```python
from build123d import *

# Parameters (mm, degrees)
DODANIE_WYCI_GNI_CIE1_DEPTH = 1.2
SZKIC3_R                    = 2.5
DODANIE_WYCI_GNI_CIE2_DEPTH = 8
SZKIC4_R                    = 1.5
WYTNIJ_WYCI_GNI_CIE1_DEPTH  = 706.226503642
SZKIC5_W                    = 5
SZKIC5_H                    = 5
DODANIE_WYCI_GNI_CIE3_DEPTH = 1
SZKIC6_W                    = 8
SZKIC6_H                    = 8
DODANIE_WYCI_GNI_CIE4_DEPTH = 3
SZKIC7_R                    = 2.5
DODANIE_WYCI_GNI_CIE5_DEPTH = 3
SZKIC8_W                    = 20.5
SZKIC8_H                    = 4
SZKIC8_H_2                  = 10
DODANIE_WYCI_GNI_CIE6_DEPTH = 2
SZKIC9_W                    = 0.66
SZKIC9_H                    = 0.66
DODANIE_WYCI_GNI_CIE7_DEPTH = 6
SZYK_LINIOWY1_COUNT         = 8
SZYK_LINIOWY1_PITCH         = 2.54
SZKIC10_W                   = 10
SZKIC10_H                   = 12
SZKIC10_W_2                 = 5
DODANIE_WYCI_GNI_CIE8_DEPTH = 2


with BuildPart() as part:
    # Szkic2 → Dodanie-wyciągnięcie1 (new body)
    with BuildSketch(Plane(origin=(0, 566.370308932, 0), x_dir=(1, 0, 0), z_dir=(0, 1, 0))):
        Polygon((-513.826446608, 398.472881439), (-513.826446608, 383.472881439), (-419.826446608, 383.472881439), (-419.826446608, 482.972881439), (-513.826446608, 482.972881439), (-513.826446608, 454.472881439), (-438.826446608, 454.472881439), (-438.826446608, 398.472881439), align=None)
    extrude(amount=DODANIE_WYCI_GNI_CIE1_DEPTH)

    # Szkic3 → Dodanie-wyciągnięcie2 (add)
    with BuildSketch(Plane(origin=(0, 567.570308932, 0), x_dir=(1, 0, 0), z_dir=(0, 1, 0))):
        with Locations(Location((-506.326446608, 461.972881439, 0), (0, 0, 180))):
            Circle(SZKIC3_R)
        with Locations(Location((-496.326446608, 461.972881439, 0), (0, 0, 180))):
            Circle(SZKIC3_R)
        with Locations(Location((-496.326446608, 390.972881439, 0), (0, 0, 180))):
            Circle(SZKIC3_R)
        with Locations(Location((-506.326446608, 390.972881439, 0), (0, 0, 180))):
            Circle(SZKIC3_R)
    extrude(amount=DODANIE_WYCI_GNI_CIE2_DEPTH)

    # Szkic4 → Wytnij-wyciągnięcie1 (cut, through all)
    with BuildSketch(Plane(origin=(0, 567.570308932, 0), x_dir=(1, 0, 0), z_dir=(0, 1, 0))):
        with Locations(Location((-434.826446608, 401.472881439, 0), (0, 0, 180))):
            Circle(SZKIC4_R)
        with Locations(Location((-434.826446608, 451.472881439, 0), (0, 0, 180))):
            Circle(SZKIC4_R)
    extrude(amount=-WYTNIJ_WYCI_GNI_CIE1_DEPTH, mode=Mode.SUBTRACT)

    # Szkic5 → Dodanie-wyciągnięcie3 (add)
    with BuildSketch(Plane.XZ.offset(-566.370308932)):
        with Locations((-506.326446608, -475.472881439)):
            Rectangle(SZKIC5_W, SZKIC5_H)
        with Locations((-496.326446608, -475.472881439)):
            Rectangle(SZKIC5_W, SZKIC5_H)
    extrude(amount=DODANIE_WYCI_GNI_CIE3_DEPTH)

    # Szkic6 → Dodanie-wyciągnięcie4 (add)
    with BuildSketch(Plane(origin=(0, 566.370308932, 0), x_dir=(-1, 0, 0), z_dir=(0, -1, 0))):
        with Locations((479.826446608, 463.972881439)):
            Rectangle(SZKIC6_W, SZKIC6_H)
    extrude(amount=DODANIE_WYCI_GNI_CIE4_DEPTH)

    # Szkic7 → Dodanie-wyciągnięcie5 (add)
    with BuildSketch(Plane.XZ.offset(-563.370308932)):
        with Locations(Location((-479.826446608, -463.972881439, 0), (0, 0, 270))):
            Circle(SZKIC7_R)
    extrude(amount=DODANIE_WYCI_GNI_CIE5_DEPTH)

    # Szkic8 → Dodanie-wyciągnięcie6 (add)
    with BuildSketch(Plane(origin=(0, 566.370308932, 0), x_dir=(-1, 0, 0), z_dir=(0, -1, 0))):
        with Locations((478.576446608, 479.972881439)):
            Rectangle(SZKIC8_W, SZKIC8_H)
        with Locations((478.576446608, 386.472881439)):
            Rectangle(SZKIC8_W, SZKIC8_H_2)
    extrude(amount=DODANIE_WYCI_GNI_CIE6_DEPTH)

    # Szkic9 → Dodanie-wyciągnięcie7 (add)
    with BuildSketch(Plane(origin=(0, 0, -481.972881439), x_dir=(-1, 0, 0), z_dir=(0, 0, -1))):
        with Locations((487.556446608, 565.360308932)):
            Rectangle(SZKIC9_W, SZKIC9_H)
    dodanie_wyci_gni_cie7 = extrude(amount=DODANIE_WYCI_GNI_CIE7_DEPTH)

    # Szyk liniowy1: Dodanie-wyciągnięcie7 ×8
    with Locations(*[(i * SZYK_LINIOWY1_PITCH, 0, 0) for i in range(1, SZYK_LINIOWY1_COUNT)]):
        add(dodanie_wyci_gni_cie7)

    # Szkic10 → Dodanie-wyciągnięcie8 (add)
    with BuildSketch(Plane(origin=(0, 566.370308932, 0), x_dir=(-1, 0, 0), z_dir=(0, -1, 0))):
        with Locations((458.326446608, 468.972881439)):
            Rectangle(SZKIC10_W, SZKIC10_H)
        with Locations((447.326446608, 468.972881439)):
            Rectangle(SZKIC10_W_2, SZKIC10_H)
    extrude(amount=DODANIE_WYCI_GNI_CIE8_DEPTH)


solid = part.part
```
Model file for the job. Use its own axes, mm. A direction names the side the tool comes from. Coordinates: 2 decimals unless noted, no trailing zeros. Loops run counter-clockwise (first coordinate to the right, second up) from the corner with the lowest first, then second, coordinate; pieces in that order, holes last. Notation, with made-up numbers: (-4, 61) - (29, 61) arc R22 ccw to (29, 85) - close; hole circle Ø10 at (-25, 31). An arc over 180 degrees is marked (long way). Answer as a JSON object with one key per item and string values. Group by question number.
(1) Cut at A-A (x = -458). Give the cut face in (y, z).
(2) Cut at D-D (x = -505). Give the cut face in (y, z), then the cut area to 3 significant figures.
(3) Two-plate mould, pull along Z, no slides. Class faces 1 (the face through (-478, 564.37, -480)), 2 (the face through (-497.48, 571.51, -464.19)), 3 (the face through (-480, 565, -459.973)), 4 (the face through (-481.35, 561.89, -461.99)): released by +Z, released by -Z, zero draft, split by the parting line, or undercut.
(4) Tool access for faces 5 (the face through (-496, 565.37, -475)), 6 (the face through (-483.826, 565, -464)), 7 (the face through (-475.826, 565, -464)), 8 (the face through (-497.48, 571.51, -393.19)), 9 (the face through (-458, 564.37, -469)): list every direction of +Z, -Z, +X, -X, +Y, -Y with a clear straight run to the whole face (end or side of a thin tool).
(5) Cut at B-B (z = -469.5). Give the cut face in (x, y), then the cut area to 3 significant figures.
(6) Probe line 1 along Z through (x, y) = (-504, 566.5); line 2 along Y through (x, z) = (-428.5, -455.5); line 3 along Y through (x, z) = (-461, -472.5). List the from-to ranges inside material, lowest first.
(7) Flat gauge pins, fed straight in: pin 1 (12 mm diameter, centred on x = -464, z = -401, fed in from -Y); pin 2 (0.7 mm diameter, centred on x = -470, z = -486, fed in from +Y); pin 3 (1.5 mm diameter, centred on x = -432, y = 567, fed in from -Z); pin 4 (2.5 mm diameter, centred on x = -434.83, z = -401.47, fed in from -Y). Where does each tip first touch, or does it go through?
(8) Cut at C-C (y = 571.5). Give the cut face in (x, z).
Geometry says:
{
 "1": {"outline": "(564.37, -474.97) - (566.37, -474.97) - (566.37, -482.97) - (567.57, -482.97) - (567.57, -454.47) - (566.37, -454.47) - (566.37, -462.97) - (564.37, -462.97) - close; (566.37, -398.47) - (567.57, -398.47) - (567.57, -383.47) - (566.37, -383.47) - close"},
 "2": {"outline": "(565.37, -477.97) - (566.37, -477.97) - (566.37, -482.97) - (567.57, -482.97) - (567.57, -464.09) - (575.57, -464.09) - (575.57, -459.85) - (567.57, -459.85) - (567.57, -454.47) - (566.37, -454.47) - (566.37, -472.97) - (565.37, -472.97) - close; (566.37, -398.47) - (567.57, -398.47) - (567.57, -393.09) - (575.57, -393.09) - (575.57, -388.85) - (567.57, -388.85) - (567.57, -383.47) - (566.37, -383.47) - close", "area": "125 mm^2"},
 "3": {"face 1": "zero draft", "face 2": "undercut", "face 3": "undercut", "face 4": "split by the parting line"},
 "4": {"face 5": "+Z, -Z, -X, -Y", "face 6": "-X, -Y", "face 7": "-Y", "face 8": "+Y", "face 9": "+Z, -Z, +X, -Y"},
 "5": {"outline": "(-513.83, 566.37) - (-463.33, 566.37) - (-463.33, 564.37) - (-453.33, 564.37) - (-453.33, 566.37) - (-449.83, 566.37) - (-449.83, 564.37) - (-444.83, 564.37) - (-444.83, 566.37) - (-419.83, 566.37) - (-419.83, 567.57) - (-513.83, 567.57) - close", "area": "143 mm^2"},
 "6": {"line 1": "z = -482.97 to -454.47, -398.47 to -383.47", "line 2": "y = 566.37 to 567.57", "line 3": "y = 564.37 to 567.57"},
 "7": {"pin 1": "stops at y = 566.37", "pin 2": "stops at y = 565.69", "pin 3": "stops at z = -482.97", "pin 4": "passes through"},
 "8": {"outline": "circle Ø5 at (-506.33, -461.97); circle Ø5 at (-506.33, -390.97); circle Ø5 at (-496.33, -461.97); circle Ø5 at (-496.33, -390.97)"}
}
